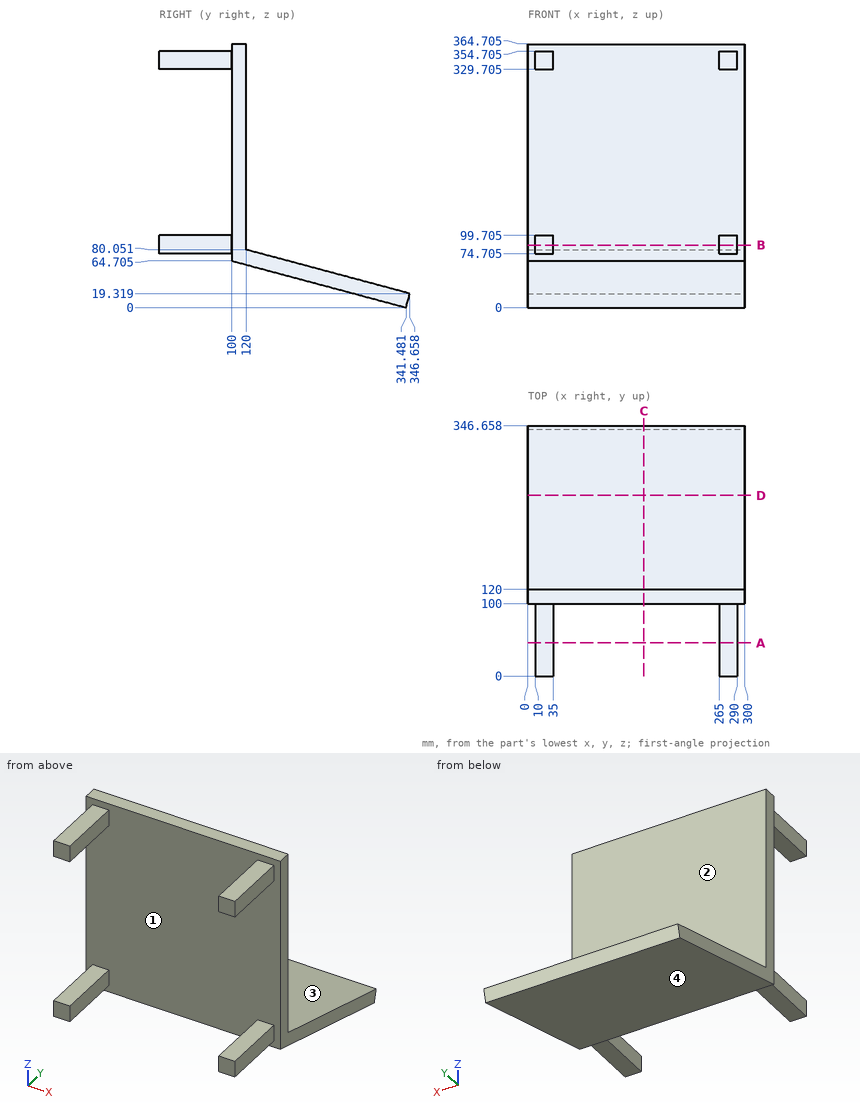
Drawing for the job (mm, zero at the part's lowest x, y, z). Give positions to 0.01 mm unless a question says otherwise; leave off trailing zeros. Loops run counter-clockwise (first coordinate to the right, second up) from the corner with the lowest first, then second, coordinate; pieces in that order, holes last.
(1) Pull direction Z, two halves, no side cores. Call the marked faces 1, 2, 3 and 4: pulls with the +Z half, pulls with the -Z half, needs draft (parallel to the pull), parting line crosses it, or undercut.
Return value:
face 1: undercut
face 2: needs draft
face 3: pulls with the +Z half
face 4: pulls with the -Z half
(2) Band-saw the part on D-D (y = 250). Write the cut outline in (x, z).
Return value:
outline: (0, 24.51) - (300, 24.51) - (300, 45.22) - (0, 45.22) - close
(3) Band-saw the part on B-B (z = 86.5). Write the cut outline in (x, y).
Return value:
outline: (0, 100) - (10, 100) - (10, 0) - (35, 0) - (35, 100) - (265, 100) - (265, 0) - (290, 0) - (290, 100) - (300, 100) - (300, 120) - (0, 120) - close
(4) Pin check, flat tips, straight feed: pin 1 (6 mm diameter, centred on x = 151.5, y = 168, fed in from +Z); pin 2 (7.5 mm diameter, centred on x = 17.5, y = 60, fed in from -Z) (1 decimal); pin 3 (12.5 mm diameter, centred on y = 55, z = 81, fed in from -X). Stop position of each tip, or through.
Return value:
pin 1: stops at z = 67.99
pin 2: stops at z = 74.7
pin 3: stops at x = 10
(5) Drill centre lines: line 1 along X through (y, z) = (31, 341.5); line 2 along Z through (x, y) = (22, 86.5) (1 decimal); line 3 along Y through (x, z) = (62, 276.5). Where is each one in solid material? Low to high.
Return value:
line 1: x = 10 to 35, 265 to 290
line 2: z = 74.7 to 99.7, 329.7 to 354.7
line 3: y = 100 to 120
(6) Band-saw the part on A-A (y = 46). Write the cut outline in (x, z) (1 decimal).
Return value:
outline: (10, 74.7) - (35, 74.7) - (35, 99.7) - (10, 99.7) - close; (10, 329.7) - (35, 329.7) - (35, 354.7) - (10, 354.7) - close; (265, 74.7) - (290, 74.7) - (290, 99.7) - (265, 99.7) - close; (265, 329.7) - (290, 329.7) - (290, 354.7) - (265, 354.7) - close
(7) Band-saw the part on C-C (x = 160.5). Write the cut outline in (y, z) (1 decimal), and give its area (3 significant figures).
Return value:
outline: (100, 64.7) - (341.5, 0) - (346.7, 19.3) - (120, 80.1) - (120, 364.7) - (100, 364.7) - close
area: 10,700 mm2
